Geometry check sheet. Reference: the model listing, model coordinates, mm. A direction names the side the tool comes from. Coordinates: 2 decimals unless noted, no trailing zeros. Write each loop counter-clockwise with the first axis right and the second up, starting at its lowest first coordinate (ties: lowest second). Pieces come first, ordered by that corner, then holes. Notation, with made-up numbers: (13.25, -14) -> (17.25, -14) arc R21 ccw to (17.25, 23) -> close; hole circle Ø8 at (56.25, -38). An arc over 180 degrees is marked (long way). One line per question, with ' | ' between items.
```python
from build123d import *

# Parameters (mm, degrees)
SKETCH1_W                      = 14
SKETCH1_H                      = 15
BOSS_EXTRUDE1_DEPTH            = 5
SKETCH3_R                      = 1.1
CUT_EXTRUDE1_DEPTH             = 14
BOSS_EXTRUDE2_DEPTH            = 4.3
SKETCH5_R                      = 1.125
CUT_EXTRUDE2_DEPTH             = 4.3
FILLET1_R                      = 2.5
CUT_EXTRUDE3_REACH             = 22.227
CUT_EXTRUDE3_DIRECTION_2_REACH = 22.227
CUT_EXTRUDE4_START             = -6
CUT_EXTRUDE4_DEPTH             = 8


with BuildPart() as part:
    # Sketch1 → Boss-Extrude1 (new body)
    with BuildSketch(Plane(origin=(0, 0, 0), x_dir=(1, 0, 0), z_dir=(0, 1, 0))):
        with Locations((0, 7.5)):
            Rectangle(SKETCH1_W, SKETCH1_H)
    extrude(amount=-BOSS_EXTRUDE1_DEPTH)

    # Sketch3 → Cut-Extrude1 (cut)
    with BuildSketch(Plane.ZY.offset(7)):
        with Locations((-12.5, -2.5)):
            Circle(SKETCH3_R)
    extrude(amount=-CUT_EXTRUDE1_DEPTH, mode=Mode.SUBTRACT)

    # Sketch4 → Boss-Extrude2 (add)
    with BuildSketch(Plane(origin=(0, 0, -15), x_dir=(-1, 0, 0), z_dir=(0, 0, -1))):
        with BuildLine():
            Line((-7, 0), (-3.763056055, 8.981248181))
            ThreePointArc((-3.763056055, 8.981248181), (0, 11.625), (3.763056055, 8.981248181))
            Line((3.763056055, 8.981248181), (7, 0))
            Line((7, 0), (-7, 0))
        make_face()
    extrude(amount=-BOSS_EXTRUDE2_DEPTH)

    # Sketch5 → Cut-Extrude2 (cut)
    with BuildSketch(Plane(origin=(0, 0, -15), x_dir=(-1, 0, 0), z_dir=(0, 0, -1))):
        with Locations((0, 7.625)):
            Circle(SKETCH5_R)
    extrude(amount=-CUT_EXTRUDE2_DEPTH, mode=Mode.SUBTRACT)

    # Fillet1
    fillet1_edges = [part.edges().sort_by_distance(p)[0] for p in [
        (0, -5, -15),
        (0, 0, -10.7),
    ]]
    fillet(fillet1_edges, radius=FILLET1_R)

    # Sketch6 → Cut-Extrude3 (cut, up to next)
    with BuildSketch(Plane(origin=(0, 0, 0), x_dir=(1, 0, 0), z_dir=(0, 1, 0)), mode=Mode.PRIVATE) as cut_extrude3_sk1:
        with BuildLine():
            Line((-3.5, -5.5), (-3.5, 5.5))
            ThreePointArc((-3.5, 5.5), (0, 9), (3.5, 5.5))
            Line((3.5, 5.5), (3.5, -5.5))
            ThreePointArc((3.5, -5.5), (0, -9), (-3.5, -5.5))
        make_face()
    cut_extrude3_tool1 = extrude(cut_extrude3_sk1.sketch, amount=-CUT_EXTRUDE3_REACH, mode=Mode.PRIVATE) & part.part
    add(cut_extrude3_tool1.solids().sort_by_distance((0, 0, 0))[0], mode=Mode.SUBTRACT)

    # Sketch6 → Cut-Extrude3 direction 2 (cut, up to next)
    with BuildSketch(Plane(origin=(0, 0, 0), x_dir=(1, 0, 0), z_dir=(0, 1, 0)), mode=Mode.PRIVATE) as cut_extrude3_direction_2_sk1:
        with BuildLine():
            Line((-3.5, -5.5), (-3.5, 5.5))
            ThreePointArc((-3.5, 5.5), (0, 9), (3.5, 5.5))
            Line((3.5, 5.5), (3.5, -5.5))
            ThreePointArc((3.5, -5.5), (0, -9), (-3.5, -5.5))
        make_face()
    cut_extrude3_direction_2_tool1 = extrude(cut_extrude3_direction_2_sk1.sketch, amount=CUT_EXTRUDE3_DIRECTION_2_REACH, mode=Mode.PRIVATE) & part.part
    add(cut_extrude3_direction_2_tool1.solids().sort_by_distance((0, 0, 0))[0], mode=Mode.SUBTRACT)

    # Mirror1: part across plane


with BuildPart() as part_1:
    add(part.part)
    add(part.part.mirror(Plane.XY))

    # Sketch10 → Cut-Extrude4 (cut)
    with BuildSketch(Plane.ZY.offset(7).offset(CUT_EXTRUDE4_START)):
        with BuildLine():
            ThreePointArc((15, -2.5), (14.267766953, -0.732233047), (12.5, 0))
            ThreePointArc((12.5, 0), (10.732233047, -0.732233047), (10, -2.5))
            ThreePointArc((10, -2.5), (10.732233047, -4.267766953), (12.5, -5))
            ThreePointArc((12.5, -5), (14.267766953, -4.267766953), (15, -2.5))
        make_face()
        with BuildLine():
            Line((15, 0), (12.5, 0))
            ThreePointArc((12.5, 0), (14.267766953, -0.732233047), (15, -2.5))
            Line((15, -2.5), (15, 0))
        make_face()
        with BuildLine():
            ThreePointArc((12.5, -5), (10.732233047, -4.267766953), (10, -2.5))
            Line((10, -2.5), (10, -5))
            Line((10, -5), (12.5, -5))
        make_face()
    extrude(amount=-CUT_EXTRUDE4_DEPTH, mode=Mode.SUBTRACT)


solid = part_1.part
```
(1) Cross-section at D-D (x = -1.75). Record the cut outline in (y, z).
Answers below:
outline: (-5, -12.5) arc R2.5 ccw to (-2.5, -15) -> (11.22, -15) -> (11.22, -10.7) -> (2.5, -10.7) arc R2.5 cw to (0.02, -8.53) -> (-5, -8.53) -> close; (-5, 8.53) -> (0.02, 8.53) arc R2.5 cw to (2.5, 10.7) -> (11.22, 10.7) -> (11.22, 15) -> (-2.5, 15) arc R2.5 ccw to (-5, 12.5) -> close; hole circle Ø2.2 at (-2.5, -12.5); hole circle Ø2.2 at (-2.5, 12.5)
(2) Draft check along Z on faces 5 (the face through (-0.098, -2.921, -11.484)), 6 (the face through (3, -4, 10)), 7 (the face through (-5, -5, 0)). Enter one of: pulls with the +Z half, pulls with the -Z half, needs draft (parallel to the pull), parting line crosses it, or undercut.
Answers below:
face 5: undercut | face 6: pulls with the +Z half | face 7: needs draft
(3) Cross-section at B-B (z = -3). Record the cut outline in (x, y), plus the area to 3 significant figures.
Answers below:
outline: (-7, -5) -> (-3.5, -5) -> (-3.5, 0) -> (-7, 0) -> close; (3.5, -5) -> (7, -5) -> (7, 0) -> (3.5, 0) -> close | area: 35.0 mm²
(4) Cross-section at C-C (z = 13.25). Record the cut outline in (x, y) (3 decimals), plus the area to 3 significant figures.
Answers below:
outline: (-7, -4.885) -> (-1, -4.885) -> (-1, -3.305) -> (-7, -3.305) -> close; (-7, -1.695) -> (-1, -1.695) -> (-1, 0) -> (7, 0) -> (3.763, 8.981) arc R4 ccw to (-3.763, 8.981) -> (-7, 0) -> close; hole circle Ø2.25 at (0, 7.625) | area: 127 mm²
(5) Cross-section at A-A (x = 0). Record the cut outline in (y, z) (3 decimals).
Answers below:
outline: (-5, -12.5) arc R2.5 ccw to (-2.5, -15) -> (6.5, -15) -> (6.5, -10.7) -> (2.5, -10.7) arc R2.5 cw to (0.131, -9) -> (-5, -9) -> close; (-5, 9) -> (0.131, 9) arc R2.5 cw to (2.5, 10.7) -> (6.5, 10.7) -> (6.5, 15) -> (0, 15) -> (0, 12.5) arc R2.5 cw to (-2.5, 10) -> (-5, 10) -> close; (8.75, -15) -> (11.625, -15) -> (11.625, -10.7) -> (8.75, -10.7) -> close; (8.75, 10.7) -> (11.625, 10.7) -> (11.625, 15) -> (8.75, 15) -> close; hole circle Ø2.2 at (-2.5, -12.5)
(6) Depth check by flat-ended pin: P1, Ø1, axis at x = 5, z = 9, coming from the +Y side; P2, Ø1, axis at y = 8.5, z = 10.5, coming from the -X side; P3, Ø0.8, axis at x = 1, z = 13.5, coming from the -Y side. Enter the tip coordinate at first touch or a pass-through.
Answers below:
P1: stops at y = 0.36 | P2: stops at x = -4.1 | P3: stops at y = 0
(7) Material ranges on line 1 (Z direction, x = -1.75, y = 5); line 2 (Z direction, x = 0.75, y = -3.25); line 3 (Y direction, x = 0, z = 12.8) (3 decimals), recorded low to high.
Answers below:
line 1: z = -15 to -10.7, 10.7 to 15 | line 2: z = -14.88 to -13.3, -11.7 to -8.92, 8.92 to 10 | line 3: y = 0 to 6.5, 8.75 to 11.625
(8) Tool access check on faces 1 (the face through (0.098, 0.752, 9.987)), 2 (the face through (-1, -2, 11)), 3 (the face through (0.098, -4.248, -14.287)), 4 (the face through (0, -2, -9)). Record the directions out of +Z, -Z, +X, -X, +Y, -Y that give a thin tool (end or side, any length) a straight path to the whole face; none if there is none.
Answers below:
face 1: +X, -X, +Y | face 2: +Z, +X, -Y | face 3: -Z, +X, -X, -Y | face 4: +Y, -Y
